The model under review builds one solid part; all positions refer to its coordinate system, in mm. Face numbers are marked on the shaded views. A direction names the side the tool comes from. Coordinates: 2 decimals unless noted, no trailing zeros. Write each loop counter-clockwise with the first axis right and the second up, starting at its lowest first coordinate (ties: lowest second). Pieces come first, ordered by that corner, then holes. Notation, with made-up numbers: (80, 3) - (121, 3) arc R5 cw to (121, 7) - close; hole circle Ø9 at (-30.75, 39.25). An arc over 180 degrees is marked (long way). Put each result on its own line as item: value.
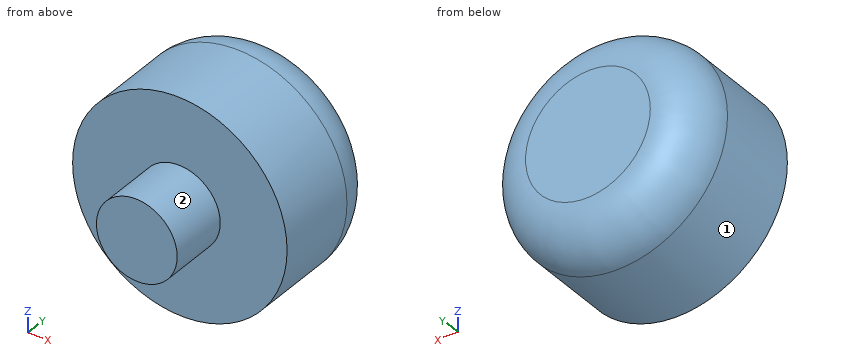
Autodesk Inventor part; units mm, degrees
ref_plane "YZ Plane" through (0, 0, 0) normal (1, 0, 0) x (0, 1, 0)
ref_plane "XZ Plane" through (0, 0, 0) normal (0, 1, 0) x (-1, 0, 0)
ref_plane "XY Plane" through (0, 0, 0) normal (0, 0, 1) x (1, 0, 0)
sketch "Sketch1" plane through (0, 0, 0) normal (0, 1, 0) x (-1, 0, 0)
  circle A0 centre (0, 0) radius 23.9
  dimension "d0" = 47.8
extrude "Extrusion1" add sketch "Sketch1" along normal blind 28.5
fillet "Fillet1" radius 10 1 edges at (23.9, 28.5, 0)
sketch "Sketch2" plane through (0, 0, 0) normal (0, -1, 0) x (1, 0, 0)
  circle A0 centre (0, 0) radius 9
  dimension "d4" = 18
extrude "Extrusion2" add sketch "Sketch2" along normal blind 13.3
thread "Thread1"
properties part number "G21.B.301111"
1. For pin 1 Ø3 at (x, z) = (12.5, -17) entering from -Y; pin 2 Ø1.5 at (y, z) = (14.5, -1.5) entering from +X; pin 3 Ø1 at (x, y) = (-18, 19.5) entering from +Z, all flat-tipped, find the tip position at first contact; note any pin that passes through.
Determined:
pin 1: stops at y = 0
pin 2: stops at x = 23.89
pin 3: stops at z = 16.21
2. Consider section A-A on z = 0. State the section outline as (x, y) points, plus the area to 3 significant figures.
Determined:
outline: (-23.9, 0) - (-9, 0) - (-9, -13.3) - (9, -13.3) - (9, 0) - (23.9, 0) - (23.9, 18.5) arc R10 ccw to (13.9, 28.5) - (-13.9, 28.5) arc R10 ccw to (-23.9, 18.5) - close
area: 1,560 mm^2
3. Consider section B-B on x = 0. State the section outline as (y, z) points, plus the area to 3 significant figures.
Determined:
outline: (-13.3, -9) - (0, -9) - (0, -23.9) - (18.5, -23.9) arc R10 ccw to (28.5, -13.9) - (28.5, 13.9) arc R10 ccw to (18.5, 23.9) - (0, 23.9) - (0, 9) - (-13.3, 9) - close
area: 1,560 mm^2
4. To check wall thickness, follow probe 1 along Y at (x, z) = (13, -3.5); probe 2 along Y at (x, z) = (11.5, -10.5); probe 3 along X at (y, z) = (8.5, -8). State the ranges of each line that lie inside material, in increasing order.
Determined:
probe 1: y = 0 to 28.5
probe 2: y = 0 to 28.36
probe 3: x = -22.52 to 22.52
5. Consider section C-C on y = -4. State the section outline as (x, z) points, plus the area to 3 significant figures.
Determined:
outline: circle Ø18 at (0, 0)
area: 254 mm^2
6. Machinability: for the marked faces 1 and 2, which of the approach directions +Z, -Z, +X, -X, +Y, -Y give a long, thin tool a straight path to every point of the face, cutting with its end or side? Answer none if there is none.
Determined:
face 1: +Y, -Y
face 2: -Y
7. Consider section D-D on y = 9. State the section outline as (x, z) points, plus the area to 3 significant figures.
Determined:
outline: circle Ø47.8 at (0, 0)
area: 1,790 mm^2
